Here's how the part is built. I have some questions about the finished solid (model axes, mm). A direction names the side the tool comes from. Give positions to 0.01 mm unless a question says otherwise; leave off trailing zeros. Loops run counter-clockwise (first coordinate to the right, second up) from the corner with the lowest first, then second, coordinate; pieces in that order, holes last. Notation, with made-up numbers: (2, 87) - (43, 87) arc R26 ccw to (43, 116) - close; hole circle Ø2 at (76.25, -19). An arc over 180 degrees is marked (long way). Put each result on its own line as item: value. Start each with the question number.
from build123d import *

# Parameters (mm, degrees)
BOSS_EXTRUDE1_DEPTH = 177.8
SKETCH2_W           = 12.7
SKETCH2_H           = 2.54
BOSS_EXTRUDE2_DEPTH = 177.8
SKETCH3_R           = 3.175
CUT_EXTRUDE1_DEPTH  = 203.727168628
SKETCH4_W           = 31.75
SKETCH4_H           = 6.35
BOSS_EXTRUDE3_DEPTH = 152.4
FILLET1_R           = 2.54


with BuildPart() as part:
    # Sketch1 → Boss-Extrude1 (new body)
    with BuildSketch(Plane(origin=(0, 0, 0), x_dir=(1, 0, 0), z_dir=(0, 1, 0))):
        Polygon((76.2, 0), (82.55, 0), (82.55, 38.1), (-82.55, 38.1), (-82.55, 0), (-76.2, 0), (-76.2, 31.75), (76.2, 31.75), align=None)
    extrude(amount=BOSS_EXTRUDE1_DEPTH)

    # Sketch2 → Boss-Extrude2 (add)
    with BuildSketch(Plane(origin=(0, 177.8, 0), x_dir=(1, 0, 0), z_dir=(0, 1, 0))):
        with Locations((88.9, 30.48)):
            Rectangle(SKETCH2_W, SKETCH2_H)
        with Locations((88.9, 21.59)):
            Rectangle(SKETCH2_W, SKETCH2_H)
        with Locations((-88.9, 21.59)):
            Rectangle(SKETCH2_W, SKETCH2_H)
        with Locations((-88.9, 30.48)):
            Rectangle(SKETCH2_W, SKETCH2_H)
    extrude(amount=-BOSS_EXTRUDE2_DEPTH)

    # Sketch3 → Cut-Extrude1 (cut, through all)
    with BuildSketch(Plane.XY.offset(-20.32)):
        with Locations((88.9, 12.7)):
            Circle(SKETCH3_R)
        with Locations((88.9, 88.9)):
            Circle(SKETCH3_R)
        with Locations((88.9, 165.1)):
            Circle(SKETCH3_R)
        with Locations((-88.9, 12.7)):
            Circle(SKETCH3_R)
        with Locations((-88.9, 165.1)):
            Circle(SKETCH3_R)
        with Locations((-88.9, 88.9)):
            Circle(SKETCH3_R)
    extrude(amount=-CUT_EXTRUDE1_DEPTH, mode=Mode.SUBTRACT)

    # Sketch4 → Boss-Extrude3 (add)
    with BuildSketch(Plane(origin=(-76.2, 0, 0), x_dir=(0, 0, -1), z_dir=(1, 0, 0))):
        with Locations((15.875, 3.175)):
            Rectangle(SKETCH4_W, SKETCH4_H)
    extrude(amount=BOSS_EXTRUDE3_DEPTH)

    # Fillet1
    fillet1_edges = [part.edges().sort_by_distance(p)[0] for p in [
        (76.2, 6.35, -15.875),
        (0, 6.35, -31.75),
        (-76.2, 6.35, -15.875),
    ]]
    fillet(fillet1_edges, radius=FILLET1_R)


solid = part.part
1) Thinking about a two-plate mould opening in Y: for faces 4 (the cylindrical face through (88.21, 85.8, -21.57)), 5 (the flat face through (-93, 90, -29.21)), 6 (the cylindrical face through (-89.59, 162, -30.46)), 7 (the flat face through (-1, 6.35, -14)), which applies, pulls with the +Y half, pulls with the -Y half, needs draft (parallel to the pull), parting line crosses it, or undercut?
2) I need wall thicknesses on line 1 (Y direction, x = 88.9, z = -21.5) (3 decimals); line 2 (X direction, y = 165.1, z = -20.85) (3 decimals); line 3 (X direction, y = 32.5, z = -19.5). Which ranges of each line are inside material? Lowest first, please.
3) Suppose I cut it at A-A on x = 88.9. Give the number of separate pieces and of enclosed holes in the cut face, plus the area to 3 significant figures.
4) Suppose I cut it at C-C on z = -13. Please give me the cut outline in (x, y).
5) I'm going to push flat-ended pins straight in: P1, Ø5.5, axis at x = -88.9, y = 165.1, coming from the -Z side; P2, Ø5, axis at y = 48, z = -35.5, coming from the -X side; P3, Ø10, axis at x = 88.9, y = 165.1, coming from the +Z side; P4, Ø4, axis at x = -89, y = 102.5, coming from the -Z side. Where does each tip first touch, or does it pass through?
6) Which directions (+Z, -Z, +X, -X, +Y, -Y) give clear straight access to the entire face, cutting with the end or side of a thin tool? Please do faces 1 (the flat face through (-93, 90, -22.86)), 2 (the flat face through (76.2, 92, -16)), 3 (the flat face through (85, 90, -31.75)).
7) Suppose I cut it at B-B on y = 115. Please give me the cut outline in (x, z).
Ans:
1. face 4: undercut
1. face 5: needs draft
1. face 6: undercut
1. face 7: pulls with the +Y half
2. line 1: y = 0 to 9.525, 15.875 to 85.725, 92.075 to 161.925, 168.275 to 177.8
2. line 2: x = -95.25 to -92.075, -85.725 to -76.2, 76.2 to 85.725, 92.075 to 95.25
2. line 3: x = -82.55 to -76.2, 76.2 to 82.55
3. separate pieces: 8
3. enclosed holes: 0
3. area: 806 mm²
4. outline: (-82.55, 0) - (82.55, 0) - (82.55, 177.8) - (76.2, 177.8) - (76.2, 8.89) arc R2.54 cw to (73.66, 6.35) - (-73.66, 6.35) arc R2.54 cw to (-76.2, 8.89) - (-76.2, 177.8) - (-82.55, 177.8) - close
5. P1: passes through
5. P2: stops at x = -82.55
5. P3: stops at z = -20.32
5. P4: stops at z = -31.75
6. face 1: -X, +Y, -Y
6. face 2: +Z, +Y
6. face 3: -Z, +X, +Y, -Y
7. outline: (-95.25, -31.75) - (-82.55, -31.75) - (-82.55, -38.1) - (82.55, -38.1) - (82.55, -31.75) - (95.25, -31.75) - (95.25, -29.21) - (82.55, -29.21) - (82.55, -22.86) - (95.25, -22.86) - (95.25, -20.32) - (82.55, -20.32) - (82.55, 0) - (76.2, 0) - (76.2, -31.75) - (-76.2, -31.75) - (-76.2, 0) - (-82.55, 0) - (-82.55, -20.32) - (-95.25, -20.32) - (-95.25, -22.86) - (-82.55, -22.86) - (-82.55, -29.21) - (-95.25, -29.21) - close
